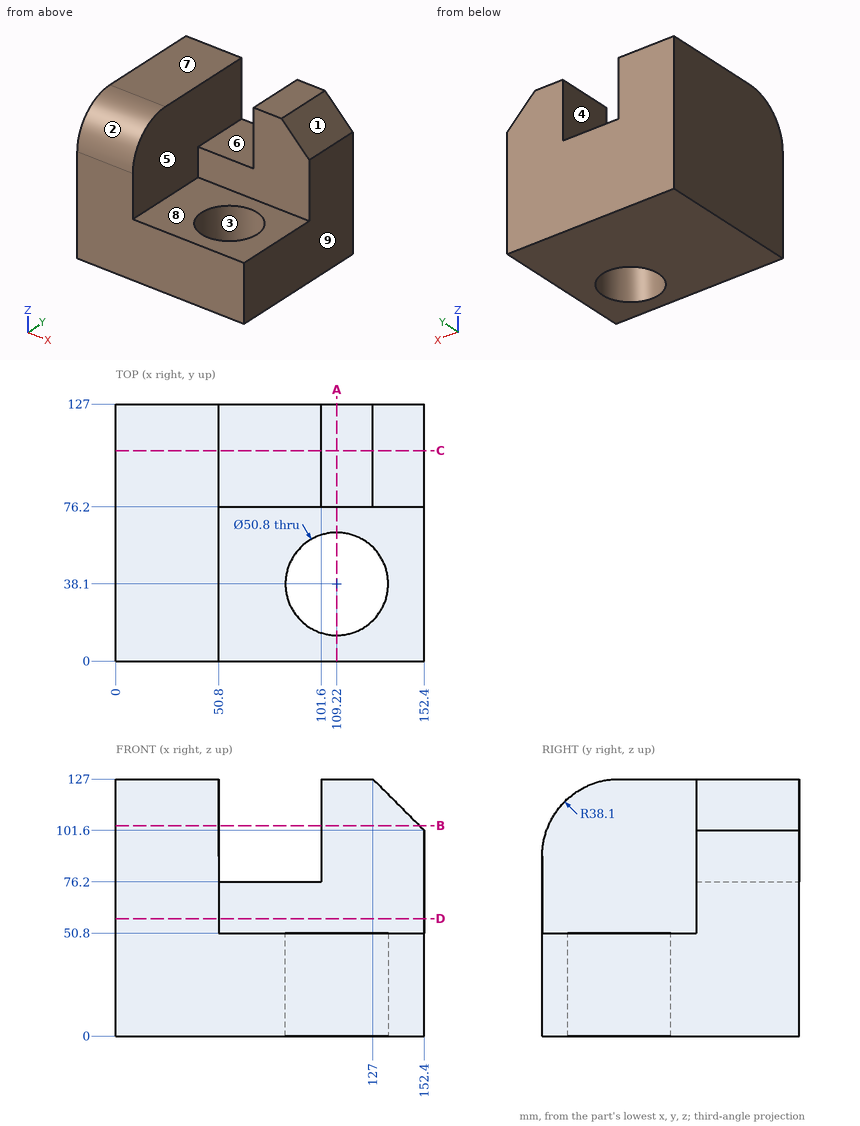
Verification items for this drawing (mm, ordinates from the low corner). A direction names the side the tool comes from. Coordinates: 2 decimals unless noted, no trailing zeros. Write each loop counter-clockwise with the first axis right and the second up, starting at its lowest first coordinate (ties: lowest second). Pieces come first, ordered by that corner, then holes. Notation, with made-up numbers: M 22.25,-35.5 L 29.25,-35.5 A20 cw 29.25,-2.5 Z; hole C 73.25,76 d2. An arc over 180 degrees is marked long. Use CSV: the item, a comma, the result in double quotes.
Q1. Section check C-C, the plane y = 104. Enter the section's corners in (x, z), and give its area (3 significant figures).
Computed values:
outline,"M 0,0 L 152.4,0 L 152.4,101.6 L 127,127 L 101.6,127 L 101.6,76.2 L 50.8,76.2 L 50.8,127 L 0,127 Z"
area,"16,500 mm²"
Q2. Section check A-A, the plane x = 109.22. Enter the section's corners in (y, z), and give its area (3 significant figures).
Computed values:
outline,"M 0,0 L 12.7,0 L 12.7,50.8 L 0,50.8 Z; M 63.5,0 L 127,0 L 127,127 L 76.2,127 L 76.2,50.8 L 63.5,50.8 Z"
area,"7,740 mm²"
Q3. Go/stop test with flat-tipped pins: P1, Ø23, axis at x = 117.5, z = 89.5, coming from the -Y side; P2, Ø1.5, axis at x = 24.5, y = 16, coming from the +Z side; P3, Ø4, axis at x = 122.5, y = 17.5, coming from the +Z side. Record where each tip stops, or that it passes through.
Computed values:
P1,"y = 76.2"
P2,"z = 120.46"
P3,"z = 50.8"
Q4. Section check B-B, the plane z = 104. Enter the section's corners in (x, y), and give its area (3 significant figures).
Computed values:
outline,"M 0,3.12 L 50.8,3.12 L 50.8,127 L 0,127 Z; M 101.6,76.2 L 150,76.2 L 150,127 L 101.6,127 Z"
area,"8,750 mm²"
Q5. Thickness scan on line 1 along X through (y, z) = (38, 20); line 2 along Y through (x, z) = (109.22, 35); line 3 along Z through (x, y) = (63.5, 111.5). Record the ranges inside material, lowest first. Write a range as [from, to].
Computed values:
line 1,"[0, 83.82], [134.62, 152.4]"
line 2,"[0, 12.7], [63.5, 127]"
line 3,"[0, 76.2]"
Q6. Section check D-D, the plane z = 58. Enter the section's corners in (x, y), and give its area (3 significant figures).
Computed values:
outline,"M 0,0 L 50.8,0 L 50.8,76.2 L 152.4,76.2 L 152.4,127 L 0,127 Z"
area,"11,600 mm²"
Q7. Mould release check, pull along X, two halves, no side actions. Record for the marked faces 1, 2, 3 and 4: pulls with the +X half, pulls with the -X half, needs draft (parallel to the pull), parting line crosses it, or undercut.
Computed values:
face 1,"pulls with the +X half"
face 2,"needs draft"
face 3,"undercut"
face 4,"undercut"
Q8. Set-up check for the marked faces 5, 6, 7, 8 and 9: record each of +Z, -Z, +X, -X, +Y, -Y from which the full face is reachable in a straight line by a thin tool's end or side.
Computed values:
face 5,"+Z, -Y"
face 6,"+Z, +Y, -Y"
face 7,"+Z, +X, -X, +Y, -Y"
face 8,"+Z, +X, -Y"
face 9,"+Z, -Z, +X, +Y, -Y"
